Geometry check sheet. Reference: the model listing, model coordinates, mm. Round coordinates to 2 decimals unless told otherwise and drop trailing zeros. Order: outer loops, then holes, each group sorted by start corner. A loop starts at its lowest first (then second) coordinate and runs counter-clockwise, first axis right, second up.
```python
from build123d import *

# Parameters (mm, degrees)
SKETCH1_R           = 4.5
BOSS_EXTRUDE2_DEPTH = 4.5
SKETCH4_OUTSIDE_W   = 42.244
SKETCH4_OUTSIDE_H   = 39.924
SKETCH4_OUTSIDE_R   = 7.5
CUT_EXTRUDE2_DEPTH  = 9
CUT_EXTRUDE2_TAPER  = 45


with BuildPart() as part:
    # Sketch1 → Boss-Extrude2 (new body, symmetric)
    with BuildSketch(Plane.XY):
        Polygon((-4.330127019, 7.5), (-8.660254038, 0), (-4.330127019, -7.5), (4.330127019, -7.5), (8.660254038, 0), (4.330127019, 7.5), align=None)
        Circle(SKETCH1_R, mode=Mode.SUBTRACT)
    extrude(amount=BOSS_EXTRUDE2_DEPTH, both=True)

    # Sketch4 outside → Cut-Extrude2 (cut)
    with BuildSketch(Plane.XY.offset(4.5)):
        Rectangle(SKETCH4_OUTSIDE_W, SKETCH4_OUTSIDE_H)
        Circle(SKETCH4_OUTSIDE_R, mode=Mode.SUBTRACT)
    cut_extrude2 = extrude(amount=-CUT_EXTRUDE2_DEPTH, taper=CUT_EXTRUDE2_TAPER, mode=Mode.SUBTRACT)

    # Mirror3: Cut-Extrude2 across plane
    add(cut_extrude2.mirror(Plane.XY), mode=Mode.SUBTRACT)


solid = part.part
```
(1) Depth check by flat-ended pin: P1, Ø1.5, axis at y = 6, z = -3, coming from the -X side; P2, Ø1, axis at x = -2.5, y = 1, coming from the -Z side; P3, Ø2, axis at y = -0.5, z = -0.5, coming from the -X side; P4, Ø3, axis at y = -5.5, z = -2.5, coming from the +X side. Enter the tip coordinate at first touch or a pass-through.
Returned:
P1: stops at x = -5.63
P2: passes through
P3: stops at x = -8.66
P4: stops at x = 6.35
(2) Sectioned sample at A-A, the plane z = 1.25. Record the cut outline in (x, y), and give its area (3 significant figures).
Returned:
outline: (-8.66, 0) - (-4.33, -7.5) - (4.33, -7.5) - (8.66, 0) - (4.33, 7.5) - (-4.33, 7.5) - close; hole circle Ø9 at (0, 0)
area: 131 mm2
(3) Material ranges on line 1 (Y direction, x = 0, z = 1); line 2 (Y direction, x = 1.75, z = -1.25); line 3 (X direction, y = -4, z = -4), recorded low to high.
Returned:
line 1: y = -7.5 to -4.5, 4.5 to 7.5
line 2: y = -7.5 to -4.15, 4.15 to 7.5
line 3: x = -6.35 to -2.06, 2.06 to 6.35
(4) Draft check along Y on faces 1 (the cylindrical face through (-0.59, 4.46, -0.06)), 2 (the flat face through (0, -5, -4.5)), 3 (the flat face through (6.526, 3.698, 0.063)). Enter one of: released by +Y, released by -Y, zero draft, split by the parting line, or undercut.
Returned:
face 1: undercut
face 2: zero draft
face 3: released by +Y
(5) Sectioned sample at B-B, the plane z = 4. Record the cut outline in (x, y), and give its area (3 significant figures).
Returned:
outline: (-7.89, -1.34) - (-5.1, -6.16) arc R8 ccw to (-2.78, -7.5) - (2.78, -7.5) arc R8 ccw to (5.1, -6.16) - (7.89, -1.34) arc R8 ccw to (7.89, 1.34) - (5.1, 6.16) arc R8 ccw to (2.78, 7.5) - (-2.78, 7.5) arc R8 ccw to (-5.1, 6.16) - (-7.89, 1.34) arc R8 ccw to start; hole circle Ø9 at (0, 0)
area: 126 mm2
